Model file for the job. Use its own axes, mm. Face numbers are marked on the shaded views. A direction names the side the tool comes from. Give positions to 0.01 mm unless a question says otherwise; leave off trailing zeros. Write each loop counter-clockwise with the first axis right and the second up, starting at its lowest first coordinate (ties: lowest second). Pieces come first, ordered by that corner, then holes. Notation, with made-up numbers: (73.5, 32) - (108.5, 32) arc R23 ccw to (108.5, 44) - close; hole circle Ø10 at (34.5, -18). An arc over 180 degrees is marked (long way). One line per item, written item: value. Start each with the question number.
(1) Cut at A-A, the plane x = -7. List the corners of the cut face in (y, z).
(2) Drop flat-ended pins along their axis: P1, Ø9, axis at x = 4, y = 27, coming from the -Z side; P2, Ø12, axis at x = 4, y = 19, coming from the +Z side; P3, Ø5, axis at x = 1.5, z = 2, coming from the +Y side; P4, Ø3, axis at y = 19, z = -1.5, coming from the -X side. Give the stop position or say it passes through.
(3) Mould opens along Y. For the marked faces 4, 5, 6 and 7 say: pulls with the +Y half, pulls with the -Y half, needs draft (parallel to the pull), parting line crosses it, or undercut.
(4) Cut at D-D, the plane x = 5.25. List the corners of the cut face in (y, z).
(5) Probe L1, parallel to Z at x = -8.25, y = 19.5; L2, parallel to X at y = 15.5, z = 2; L3, parallel to Y at x = -7.25, z = 4.75. List the from-to ranges inside material, lowest first.
(6) 3-axis set-ups, long thin cutter, end or side, ignore diameter. For the marked faces 1, 2 and 3: which of +Z, -Z, +X, -X, +Y, -Y reach the whole face in a straight line?
(7) Cut at C-C, the plane x = 0. List the corners of the cut face in (y, z), and give its area (3 significant figures).
(8) Cut at B-B, the plane z = 4. List the corners of the cut face in (x, y).
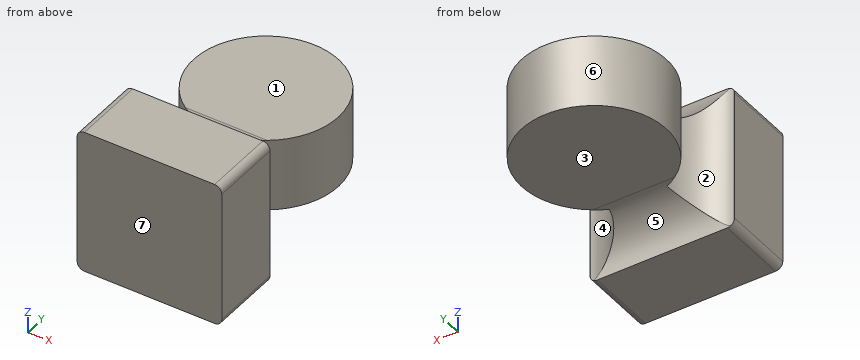
from build123d import *
from OCP.BRepAlgoAPI import BRepAlgoAPI_Cut
from OCP.TopTools import TopTools_ListOfShape

# Parameters (mm, degrees)
SKIZZE1_W                       = 20
SKIZZE1_H                       = 20
AUFSATZ_LINEAR_AUSTRAGEN1_DEPTH = 10
AUFSATZ_LINEAR_AUSTRAGEN2_DEPTH = 5
VERRUNDUNG1_START               = -5
VERRUNDUNG1_DEPTH               = 10
VERRUNDUNG1_START_2             = -10.000001186
VERRUNDUNG1_2_DEPTH             = 20.000001186
VERRUNDUNG1_START_3             = -11
VERRUNDUNG1_3_DEPTH             = 22
VERRUNDUNG2_R                   = 1


with BuildPart() as part:
    # Skizze1 → Aufsatz-Linear austragen1 (new body)
    with BuildSketch(Plane(origin=(0, 0, 0), x_dir=(1, 0, 0), z_dir=(0, 1, 0))):
        Rectangle(SKIZZE1_W, SKIZZE1_H)
    extrude(amount=AUFSATZ_LINEAR_AUSTRAGEN1_DEPTH)

    # Skizze3 → Aufsatz-Linear austragen2 (add, symmetric)
    with BuildSketch(Plane.XY):
        with BuildLine():
            Line((-4, 15), (-4, 10))
            Line((-4, 10), (4, 10))
            Line((4, 10), (4, 15))
            ThreePointArc((4, 15), (0, 34.16515139), (-4, 15))
        make_face()
    extrude(amount=AUFSATZ_LINEAR_AUSTRAGEN2_DEPTH, both=True)


with BuildPart() as verrundung1_tool:
    # Verrundung1: read off the stored shape, not the designer's step
    # Verrundung1 outline → Verrundung1 (new body)
    with BuildSketch(Plane.XY.offset(VERRUNDUNG1_START)):
        with BuildLine():
            Line((4, 10), (9.916079783, 10))
            ThreePointArc((9.916079783, 10), (6.043096437, 11.417424305), (4, 15))
            Line((4, 15), (4, 10))
        make_face()
        with BuildLine():
            Line((-9.916079783, 10), (-4, 10))
            Line((-4, 10), (-4, 15))
            ThreePointArc((-4, 15), (-6.043096437, 11.417424305), (-9.916079783, 10))
        make_face()
    extrude(amount=VERRUNDUNG1_DEPTH)


with BuildPart() as part_1:
    add(part.part)


with BuildPart() as part_2:
    # Verrundung1: joined with verrundung1_tool
    add(part_1.part.fuse(verrundung1_tool.part, tol=0.00001))


with BuildPart() as verrundung1_2_tool:
    # Verrundung1 2 outline → Verrundung1 2 (new body)
    with BuildSketch(Plane.XY.offset(VERRUNDUNG1_START_2)):
        with BuildLine():
            Line((-9.916079783, 10), (9.916079783, 10))
            ThreePointArc((9.916079783, 10), (6.043096437, 11.417424305), (4, 15))
            ThreePointArc((4, 15), (0, 34.16515139), (-4, 15))
            ThreePointArc((-4, 15), (-6.043096437, 11.417424305), (-9.916079783, 10))
        make_face()
    extrude(amount=VERRUNDUNG1_2_DEPTH)


with BuildPart() as part_3:
    add(part_2.part)


with BuildPart() as part_4:
    # Verrundung1 2: joined with verrundung1_2_tool
    add(part_3.part.fuse(verrundung1_2_tool.part, tol=0.00001))


with BuildPart() as verrundung1_3_tool:
    # Verrundung1 3 outline → Verrundung1 3 (new body)
    with BuildSketch(Plane.YZ.offset(VERRUNDUNG1_START_3)):
        with BuildLine():
            Line((15.916079783, 5), (34.16515139, 5))
            Line((34.16515139, 5), (36, 5))
            Line((36, 5), (36, 10))
            Line((36, 10), (34.16515139, 10))
            Line((34.16515139, 10), (9.999989402, 10.000062699))
            ThreePointArc((9.999989402, 10.000062699), (12.043072154, 6.417444828), (15.916079783, 5))
        make_face()
        with BuildLine():
            Line((36, -10.000001186), (36, -5))
            Line((36, -5), (34.16515139, -5))
            Line((34.16515139, -5), (15.916079783, -5))
            ThreePointArc((15.916079783, -5), (12.043072154, -6.417444828), (9.999989402, -10.000062699))
            Line((9.999989402, -10.000062699), (34.16515139, -10.000001186))
            Line((34.16515139, -10.000001186), (36, -10.000001186))
        make_face()
    extrude(amount=VERRUNDUNG1_3_DEPTH)


with BuildPart() as part_5:
    add(part_4.part)

    # Verrundung1 3: cut by verrundung1_3_tool, with a tolerance
    verrundung1_3_stock = TopTools_ListOfShape()
    verrundung1_3_stock.Append(part_5.part.wrapped)
    verrundung1_3_tools = TopTools_ListOfShape()
    verrundung1_3_tools.Append(verrundung1_3_tool.part.wrapped)
    verrundung1_3_cut = BRepAlgoAPI_Cut()
    verrundung1_3_cut.SetArguments(verrundung1_3_stock)
    verrundung1_3_cut.SetTools(verrundung1_3_tools)
    verrundung1_3_cut.SetFuzzyValue(0.00001)
    verrundung1_3_cut.Build()
    add(Compound.cast(verrundung1_3_cut.Shape()).solids(), mode=Mode.REPLACE)

    # Verrundung2
    # the kernel refuses this fillet: 1 mm, written as the material it takes off along each edge
    with BuildSketch(Plane(origin=(-10, -2.5, 10), x_dir=(1, 0, 0), z_dir=(0, 1, 0)), Plane(origin=(-10, -2.5, -10), x_dir=(0, 0, 1), z_dir=(0, 1, 0))) as verrundung2_piece_1:
        with BuildLine():
            CenterArc((VERRUNDUNG2_R, VERRUNDUNG2_R), VERRUNDUNG2_R, 180, 90)
            Line((0, VERRUNDUNG2_R), (0, 0))
            Line((0, 0), (VERRUNDUNG2_R, 0))
        make_face()
    extrude(amount=15, mode=Mode.SUBTRACT)
    with BuildSketch(Plane(origin=(10, -2.5, -10), x_dir=(0, 0, 1), z_dir=(0, 1, 0)), Plane(origin=(10, -2.5, 10), x_dir=(-1, 0, 0), z_dir=(0, 1, 0))) as verrundung2_piece_2:
        with BuildLine():
            CenterArc((VERRUNDUNG2_R, -VERRUNDUNG2_R), VERRUNDUNG2_R, 90, 90)
            Line((0, -VERRUNDUNG2_R), (0, 0))
            Line((0, 0), (VERRUNDUNG2_R, 0))
        make_face()
    extrude(amount=15, mode=Mode.SUBTRACT)


solid = part_5.part
Answers follow:
1. outline: (0, -10) - (10, -10) arc R6 cw to (10.76, -7.94) - (10.76, 7.94) arc R6 cw to (10, 10) - (0, 10) - close; (17.02, -5) - (31.31, -5) - (31.31, 5) - (17.02, 5) - close
2. P1: stops at z = -5
2. P2: stops at z = 5.76
2. P3: stops at y = 34.17
2. P4: stops at x = -9.3
3. face 4: undercut
3. face 5: pulls with the +Y half
3. face 6: undercut
3. face 7: pulls with the -Y half
4. outline: (0, -10) - (10, -10) arc R6 cw to (12.23, -6.27) - (12.23, 6.27) arc R6 cw to (10, 10) - (0, 10) - close; (15.65, -5.01) arc R6 cw to (15.92, -5) - (32.68, -5) - (32.68, 5) - (15.92, 5) arc R6 cw to (15.65, 5.01) - close
5. L1: z = -5 to 5
5. L2: x = -4.99 to 4.99
5. L3: y = 0 to 10.62, 17.28 to 31.05
6. face 1: +Z, +X, -X, +Y
6. face 2: +Z, -Z, -X
6. face 3: -Z, +X, -X, +Y
7. outline: (0, -10) - (10, -10) arc R6 cw to (15.92, -5) - (34.17, -5) - (34.17, 5) - (15.92, 5) arc R6 cw to (10, 10) - (0, 10) - close
7. area: 456 mm²
8. outline: (-10, 0) - (10, 0) - (10, 10) - (9.92, 10) arc R6 cw to (4, 15) arc R10 ccw (long way) to (-4, 15) arc R6 cw to (-9.92, 10) - (-10, 10) - close
